from build123d import *

# Parameters (mm, degrees)
F0_R     = 3
F1_DEPTH = 150
F0_R_2   = 7.4761454261
F2_DEPTH = 155
F0_R_3   = 27
F3_DEPTH = 150


with BuildPart() as f1:
    # F0 (on Front) → F1 (new body, symmetric)
    with BuildSketch(Plane.XZ):
        Circle(F0_R)
    extrude(amount=F1_DEPTH, both=True)

    # F0 (on Front) → F2 (join, symmetric)
    with BuildSketch(Plane.XZ):
        Circle(F0_R_2)
        Circle(F0_R, mode=Mode.SUBTRACT)
    extrude(amount=F2_DEPTH, both=True)

    # F0 (on Front) → F3 (join, symmetric)
    with BuildSketch(Plane.XZ):
        Circle(F0_R_3)
        Circle(F0_R_2, mode=Mode.SUBTRACT)
    extrude(amount=F3_DEPTH, both=True)


solid = f1.part
Geometry check sheet. Reference: the model listing, model coordinates, mm. A direction names the side the tool comes from. Round coordinates to 2 decimals unless told otherwise and drop trailing zeros. Order: outer loops, then holes, each group sorted by start corner. A loop starts at its lowest first (then second) coordinate and runs counter-clockwise, first axis right, second up. Notation, with made-up numbers: (-15.75, 64.25) - (24.25, 64.25) arc R21 ccw to (24.25, 101.25) - close; hole circle Ø10 at (39.5, 57.5). An arc over 180 degrees is marked (long way). One line per question, with ' | ' between items. Start each with the question number.
(1) Access from +Z, -Z, +X, -X, +Y, -Y to the whole of each face (thin tool, end or side, straight path). Record for faces 1 (the cylindrical face through (3.45, 152.465, -6.633)), 2 (the cylindrical face through (-5.85, -2.1, -26.36)), 3 (the cylindrical face through (-3, -152, 0)).
(2) Sectioned sample at C-C on y = -11. Record the cut outline in (x, z).
(3) Release check for a two-part mould opening along Z. For faces 4 (the cylindrical face through (3.45, -152.535, -6.633)), 5 (the flat face through (0, 150, 0)), 6 (the flat face through (6, -150, -6)), 7 (the flat face through (0, -150, 0)) record: released by +Z, released by -Z, zero draft, split by the parting line, or undercut.
(4) Sectioned sample at A-A on x = 0. Record the cut outline in (y, z).
(5) Depth check by flat-ended pin: pin 1 Ø3.5 at (x, z) = (0, 0) entering from +Y; pin 2 Ø6 at (x, y) = (-13, 53) entering from +Z; pin 3 Ø2 at (x, z) = (-20.5, -19) entering from -Y. Enter the tip coordinate at first touch or a pass-through.
(6) Sectioned sample at D-D on z = -21.5. Record the cut outline in (x, y).
(7) Sectioned sample at B-B on z = 0. Record the cut outline in (x, y).
(8) Thickness scan on L1, parallel to Z at x = 0, y = -152.8; L2, parallel to Y at x = 11, z = 11; L3, parallel to Z at x = 0, y = -23.5. Record the ranges inside material, lowest first. Write a range as [from, to].
Conclusion:
1) face 1: +Y | face 2: +Y, -Y | face 3: -Y
2) outline: circle Ø54 at (0, 0)
3) face 4: split by the parting line | face 5: undercut | face 6: zero draft | face 7: undercut
4) outline: (-155, -7.48) - (-150, -7.48) - (-150, -27) - (150, -27) - (150, -7.48) - (155, -7.48) - (155, -3) - (150, -3) - (150, 3) - (155, 3) - (155, 7.48) - (150, 7.48) - (150, 27) - (-150, 27) - (-150, 7.48) - (-155, 7.48) - (-155, 3) - (-150, 3) - (-150, -3) - (-155, -3) - close
5) pin 1: stops at y = 150 | pin 2: stops at z = 25.08 | pin 3: stops at y = -150
6) outline: (-16.33, -150) - (16.33, -150) - (16.33, 150) - (-16.33, 150) - close
7) outline: (-27, -150) - (-7.48, -150) - (-7.48, -155) - (-3, -155) - (-3, -150) - (3, -150) - (3, -155) - (7.48, -155) - (7.48, -150) - (27, -150) - (27, 150) - (7.48, 150) - (7.48, 155) - (3, 155) - (3, 150) - (-3, 150) - (-3, 155) - (-7.48, 155) - (-7.48, 150) - (-27, 150) - close
8) L1: z = [-7.48, -3], [3, 7.48] | L2: y = [-150, 150] | L3: z = [-27, 27]
